Read the model definition and answer for the solid it produces. Units are mm, in the model's axes. A direction names the side the tool comes from. Give positions to 0.01 mm unless a question says otherwise; leave off trailing zeros. Loops run counter-clockwise (first coordinate to the right, second up) from the corner with the lowest first, then second, coordinate; pieces in that order, holes last.
(1) Find section B-B, the plane y = -5.5. Write down the section's boundary in (x, z).
(2) Each of these flat-tipped pins is pushed along its axis until it touches: P1, Ø6, axis at y = 10.5, z = 31, coming from the -X side; P2, Ø8, axis at x = 15.5, z = 34.5, coming from the -Y side; P3, Ø5, axis at x = -3.91, y = -0.86, coming from the +Z side; P4, Ø2, axis at y = 14.5, z = 18, coming from the +X side. Where does it stop, or does it pass through?
(3) Determine the mould class of faces 1 (the face through (28.606, -12.188, 20.854)), 2 (the face through (4, 9, 0)), 3 (the face through (18.284, 11.304, 20.854)), 4 (the face through (-3.807, -4.856, 20.854)) for opening direction Y: pulls with the +Y half, pulls with the -Y half, needs draft (parallel to the pull), parting line crosses it, or undercut.
(4) Straight lines are drawn through the part: probe 1 along X at (y, z) = (-2.5, 30.5); probe 2 along X at (y, z) = (17.5, 17); probe 3 along X at (y, z) = (8.5, 14). For each, find the intervals that lie inside material, in ascending order.
(5) Find section A-A, the plane z = 10. Write down the section's boundary in (x, y), then the cut area to 3 significant figures.
(6) Which of the six approach directions +Z, -Z, +X, -X, +Y, -Y give full straight-line access (tool end or side, diameter ignored) to faces 5 (the face through (3, 34.7, 21)), 6 (the face through (-10, 0, 21))?
(7) Find section C-C, the plane x = 27. Write down the section's boundary in (y, z), then the cut area to 3 significant figures.
(8) Find section D-D, the plane y = 9. Write down the section's boundary in (x, z), then the cut area to 3 significant figures.
```python
from build123d import *

# Parameters (mm, degrees)
F3_DEPTH = 42.3
F4_W     = 5.0520027294
F4_H     = 42.3
F5_DEPTH = 34.7
F7_DEPTH = 42.3


# Not quite as in the source:
# - the program builds the solid bodies; features that only make, move or delete a surface that nothing else refers to are left out


with BuildPart() as f3:
    # F0 (on Top) → F3 (new body)
    with BuildSketch(Plane.XY):
        with BuildLine():
            ThreePointArc((0, 0), (-3.9070909635, -4.8571115465), (-7.8141819269, 0))
            Line((-7.8141819269, 0), (-12.8661846563, 0))
            ThreePointArc((-12.8661846563, 0), (-3.9070909635, -9.8571115465), (5.0520027294, 0))
            Line((5.0520027294, 0), (0, 0))
        make_face()
    extrude(amount=F3_DEPTH)

    # F4 (on face) → F5 (join)
    with BuildSketch(Plane(origin=(0, 0, 0), x_dir=(-1, 0, 0), z_dir=(0, 1, 0))):
        with Locations((-2.5260013647, 21.15)):
            Rectangle(F4_W, F4_H)
    extrude(amount=F5_DEPTH)

    # F6 (on Top) → F7 (join)
    with BuildSketch(Plane.XY):
        Polygon((31.1498828232, -10.7009746134), (4.7412305139, 34.4645157456), (4.6712128018, 23.0707097992), (26.133000959, -13.6343887705), align=None)
    extrude(amount=F7_DEPTH)


solid = f3.part
```
Entries:
1. outline: (-11.62, 0) - (3.8, 0) - (3.8, 42.3) - (-11.62, 42.3) - close; (21.38, 0) - (28.11, 0) - (28.11, 42.3) - (21.38, 42.3) - close
2. P1: stops at x = 0
2. P2: stops at y = -2.29
2. P3: passes through
2. P4: stops at x = 17
3. face 1: pulls with the -Y half
3. face 2: needs draft
3. face 3: pulls with the +Y half
3. face 4: undercut
4. probe 1: x = -12.76 to -7.55, -0.26 to 4.94, 19.62 to 26.35
4. probe 2: x = 0 to 5.05, 7.93 to 14.66
4. probe 3: x = 0 to 5.05, 13.19 to 19.92
5. outline: (-12.87, 0) arc R9 ccw (long way) to (5.05, 0) - (5.05, 22.42) - (26.13, -13.63) - (31.15, -10.7) - (5.05, 33.93) - (5.05, 34.7) - (0, 34.7) - (0, 0) arc R4 cw (long way) to (-7.81, 0) - close
5. area: 558 mm2
6. face 5: +Z, -Z, +X, -X, +Y
6. face 6: +Z, -Z, -X, +Y
7. outline: (-13.13, 0) - (-3.6, 0) - (-3.6, 42.3) - (-13.13, 42.3) - close
7. area: 403 mm2
8. outline: (0, 0) - (5.05, 0) - (5.05, 42.3) - (0, 42.3) - close; (12.9, 0) - (19.63, 0) - (19.63, 42.3) - (12.9, 42.3) - close
8. area: 498 mm2
